Autodesk Inventor part; units mm, degrees
ref_plane "YZ Plane" through (0, 0, 0) normal (1, 0, 0) x (0, 1, 0)
ref_plane "XZ Plane" through (0, 0, 0) normal (0, 1, 0) x (-1, 0, 0)
ref_plane "XY Plane" through (0, 0, 0) normal (0, 0, 1) x (1, 0, 0)
sketch "Boceto1" plane through (0, 0, 0) normal (0, 1, 0) x (-1, 0, 0)
  circle A0 centre (0, -16) radius 2
  circle A1 centre (13.856406, -8) radius 2
  circle A2 centre (13.856406, 8) radius 2
  circle A3 centre (0, 16) radius 2
  circle A4 centre (-13.856406, 8) radius 2
  circle A5 centre (-13.856406, -8) radius 2
  line L0 (-12.759095, -9.672097) -> (-5.490746, -5.928235)
  line L1 (-6.410449, -1.764863) -> (-14.746933, -6.209201)
  line L2 (-6.410449, 1.764863) -> (-14.746933, 6.209201)
  line L3 (-12.759095, 9.672097) -> (-5.490746, 5.928235)
  line L4 (2, 16) -> (2.583184, 7.574131)
  line L5 (-2, 16) -> (-2.579628, 7.569051)
  line L6 (2.579349, -7.573106) -> (2, -16)
  line L7 (-2.579628, -7.569051) -> (-2, -16)
  line L8 (12.856406, 9.732051) -> (5.495313, 5.934789)
  line L9 (14.856406, 6.267949) -> (6.4102, 1.764839)
  line L10 (14.856406, -6.267949) -> (6.4102, -1.764839)
  line L11 (12.856406, -9.732051) -> (5.491541, -5.932843)
  circle A6 centre (0, 0) radius 3
  arc A7 (-6.410449, -1.764863) -> (-6.410449, 1.764863) centre (-7.351331, 0) ccw
  arc A8 (-2.579628, -7.569051) -> (-5.490746, -5.928235) centre (-4.574918, -7.706228) ccw
  arc A9 (5.491541, -5.932843) -> (2.579349, -7.573106) centre (4.574639, -7.710282) ccw
  arc A10 (6.4102, 1.764839) -> (6.4102, -1.764839) centre (7.351127, 0) ccw
  arc A11 (2.583184, 7.574131) -> (5.495313, 5.934789) centre (4.578411, 7.712228) ccw
  arc A12 (-5.490746, 5.928235) -> (-2.579628, 7.569051) centre (-4.574918, 7.706228) ccw
  point P0 (0, -3.1)
  point P1 (-3.1, 0)
  point P2 (0, 3.1)
  point P3 (3.1, 0)
  dimension "d17" = 360
  dimension "d19" = 6
  dimension "d20" = 2
sketch "Boceto1 outline for Extrusión1" plane through (0, 0, 0) normal (0, 1, 0) x (-1, 0, 0)
  arc A0 (5.495313, 5.934789) -> (2.583184, 7.574131) centre (4.578411, 7.712228) cw
  line L0 (12.856406, 9.732051) -> (5.495313, 5.934789)
  line L1 (2.583184, 7.574131) -> (2, 16)
  arc A1 (14.856406, 6.267949) -> (12.856406, 9.732051) centre (13.856406, 8) ccw
  arc A2 (2, 16) -> (-2, 16) centre (0, 16) ccw
  line L2 (6.4102, 1.764839) -> (14.856406, 6.267949)
  line L3 (-2, 16) -> (-2.579628, 7.569051)
  arc A3 (6.4102, -1.764839) -> (6.4102, 1.764839) centre (7.351127, 0) cw
  arc A4 (-2.579628, 7.569051) -> (-5.490746, 5.928235) centre (-4.574918, 7.706228) cw
  line L4 (14.856406, -6.267949) -> (6.4102, -1.764839)
  line L5 (-5.490746, 5.928235) -> (-12.759095, 9.672097)
  arc A5 (12.856406, -9.732051) -> (14.856406, -6.267949) centre (13.856406, -8) ccw
  arc A6 (-12.759095, 9.672097) -> (-14.746933, 6.209201) centre (-13.856406, 8) ccw
  line L6 (5.491541, -5.932843) -> (12.856406, -9.732051)
  line L7 (-14.746933, 6.209201) -> (-6.410449, 1.764863)
  arc A7 (2.579349, -7.573106) -> (5.491541, -5.932843) centre (4.574639, -7.710282) cw
  arc A8 (-6.410449, 1.764863) -> (-6.410449, -1.764863) centre (-7.351331, 0) cw
  line L8 (2, -16) -> (2.579349, -7.573106)
  line L9 (-6.410449, -1.764863) -> (-14.746933, -6.209201)
  arc A9 (-2, -16) -> (2, -16) centre (0, -16) ccw
  arc A10 (-14.746933, -6.209201) -> (-12.759095, -9.672097) centre (-13.856406, -8) ccw
  line L10 (-2.579628, -7.569051) -> (-2, -16)
  line L11 (-12.759095, -9.672097) -> (-5.490746, -5.928235)
  arc A11 (-5.490746, -5.928235) -> (-2.579628, -7.569051) centre (-4.574918, -7.706228) cw
  circle A12 centre (0, 0) radius 3
extrude "Extrusión1" add sketch "Boceto1 outline for Extrusión1" along normal blind 3
sketch "Boceto2" plane through (0, 3, 0) normal (0, 1, 0) x (1, 0, 0)
  arc A0 (-14.856406, -6.267949) -> (-12.856406, -9.732051) centre (-13.856406, -8) ccw
  circle A1 centre (-13.856406, -8) radius 1.25
  arc A2 (-2, -16) -> (2, -16) centre (0, -16) ccw
  circle A3 centre (0, -16) radius 1.25
  arc A4 (-12.856406, 9.732051) -> (-14.856406, 6.267949) centre (-13.856406, 8) ccw
  circle A5 centre (-13.856406, 8) radius 1.25
  arc A6 (2, 16) -> (-2, 16) centre (0, 16) ccw
  circle A7 centre (0, 16) radius 1.25
  arc A8 (14.746933, 6.209201) -> (12.759095, 9.672097) centre (13.856406, 8) ccw
  circle A9 centre (13.856406, 8) radius 1.25
  arc A10 (12.759095, -9.672097) -> (14.746933, -6.209201) centre (13.856406, -8) ccw
  circle A11 centre (13.856406, -8) radius 1.25
  point P0 (0, 0)
  dimension "d23" = 2.5
  dimension "d24" = 2.5
  dimension "d25" = 2.5
  dimension "d26" = 2.5
  dimension "d27" = 2.5
  dimension "d28" = 2.5
hole "Agujero1" at (0, 3, -16) at (-13.856406, 3, -8) at (0, 3, 16) at (13.856406, 3, 8) at (13.856406, 3, -8) direction (0, -1, 0) diameter 2.5 end through all
sketch "Boceto3" plane through (0, 3, 0) normal (0, 1, 0) x (1, 0, 0)
  arc A0 (-14.856406, -6.267949) -> (-12.856406, -9.732051) centre (-13.856406, -8) ccw
  circle A1 centre (-13.856406, -8) radius 1.25
  point P0 (0, 0)
  dimension "d36" = 2.5
hole "Agujero2" at (-13.856406, 3, 8) direction (0, -1, 0) diameter 2.5 end through all
sketch "Boceto4" plane through (0, 3, 0) normal (0, 1, 0) x (1, 0, 0)
  point P0 (0, 0)
properties part number "Extension"
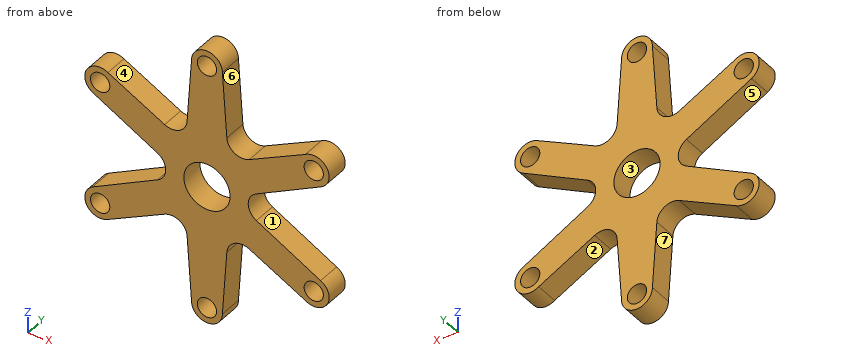
Verification items for the finished model (mm, model axes). Face numbers are marked on the shaded views. A direction names the side the tool comes from. Coordinates: 2 decimals unless noted, no trailing zeros. Write each loop counter-clockwise with the first axis right and the second up, starting at its lowest first coordinate (ties: lowest second). Pieces come first, ordered by that corner, then holes. Notation, with made-up numbers: M 12.5,37 L 17.5,37 A13 cw 17.5,52 Z; hole C 61,39.5 d1. An arc over 180 degrees is marked long. Answer as a JSON object with one key per item and string values. Group by question number.
(1) Cross-section at B-B, the plane z = 0. Record the cut outline in (x, y), and give its area (3 significant figures).
(2) Tool access check on the marked faces 5, 6 and 7. Record the directions out of +Z, -Z, +X, -X, +Y, -Y that give a thin tool (end or side, any length) a straight path to the whole face; none if there is none.
(3) Material ranges on line 1 (Z direction, x = 0, y = 2.3); line 2 (X direction, y = 1.25, z = 6.5); line 3 (X direction, y = 1.45, z = 8), recorded low to high.
(4) Cross-section at A-A, the plane x = 0. Record the cut outline in (y, z), and give its area (3 significant figures).
(5) Release check for a two-part mould opening along Z. For the marked faces 1, 2, 3 and 4 record: +Z half, -Z half, draft (parallel to the pull), parting line (faces both ways), or undercut.
(6) Cross-section at C-C, the plane x = -10.5. Record the cut outline in (y, z), and give its area (3 significant figures).
(7) Cross-section at D-D, the plane z = 8. Record the cut outline in (x, y).
(8) Gauge pin test, flat ends, axial feed: pin 1 (6 mm diameter, centred on x = 6.5, z = -14, fed in from +Y); pin 2 (1 mm diameter, centred on y = 2, z = 9.5, fed in from -X). Record the tip position at first contact, or that the pin passes through.
Reply:
{
 "1": {"outline": "M -5.35,0 L -3,0 L -3,3 L -5.35,3 Z; M 3,0 L 5.35,0 L 5.35,3 L 3,3 Z", "area": "14.1 mm²"},
 "2": {"face 5": "-X, +Y, -Y", "face 6": "+Z, +Y, -Y", "face 7": "-Z, +Y, -Y"},
 "3": {"line 1": "-18 to -17.25, -14.75 to -3, 3 to 14.75, 17.25 to 18", "line 2": "-15.18 to -6.59, -2.99 to 2.98, 6.6 to 15.18", "line 3": "-15.86 to -15.11, -12.61 to -9.5, -2.55 to 2.55, 9.51 to 12.61, 15.11 to 15.86"},
 "4": {"outline": "M 0,-18 L 3,-18 L 3,-17.25 L 0,-17.25 Z; M 0,-14.75 L 3,-14.75 L 3,-3 L 0,-3 Z; M 0,3 L 3,3 L 3,14.75 L 0,14.75 Z; M 0,17.25 L 3,17.25 L 3,18 L 0,18 Z", "area": "75.0 mm²"},
 "5": {"face 1": "undercut", "face 2": "-Z half", "face 3": "undercut", "face 4": "+Z half"},
 "6": {"outline": "M 0,-8.52 L 3,-8.52 L 3,-3.95 L 0,-3.95 Z; M 0,3.95 L 3,3.95 L 3,8.52 L 0,8.52 Z", "area": "27.4 mm²"},
 "7": {"outline": "M -15.86,0 L -15.11,0 L -15.11,3 L -15.86,3 Z; M -12.61,0 L -9.5,0 L -9.5,3 L -12.61,3 Z; M -2.55,0 L 2.55,0 L 2.55,3 L -2.55,3 Z; M 9.51,0 L 12.61,0 L 12.61,3 L 9.51,3 Z; M 15.11,0 L 15.86,0 L 15.86,3 L 15.11,3 Z"},
 "8": {"pin 1": "through", "pin 2": "x = -15.59"}
}
